```python
from build123d import *

# Parameters (mm, degrees)
SKETCH_4_OUTSIDE_W        = 310.112
SKETCH_4_OUTSIDE_H        = 310.112
CUT_EXTRUDE_1_DEPTH       = 28
HOLE_WIZARD_1_D           = 9
HOLE_WIZARD_1_CBORE_D     = 15
HOLE_WIZARD_1_CBORE_DEPTH = 9
HOLE_WIZARD_M30_2_D       = 26.5
CHAMFER_1_SIZE            = 1


with BuildPart() as part:
    # 草图3 → 旋转1 (revolve)
    with BuildSketch(Plane.XY, mode=Mode.PRIVATE) as revolve_1_sk:
        Polygon((0, 0), (-28, 0), (-28, -4), (-40, -4), (-80, -12), (-120, -12), (-120, -28), (-81, -28), (-45, -24), (0, -24), align=None)
    revolve(revolve_1_sk.sketch.rotate(Axis((0, 0, 0), (0, -1, 0)), 270), axis=Axis((0, 0, 0), (0, -1, 0)))

    # 草图4 outside → 切除-拉伸1 (cut)
    with BuildSketch(Plane(origin=(0, 0, 0), x_dir=(1, 0, 0), z_dir=(0, 1, 0))):
        Rectangle(SKETCH_4_OUTSIDE_W, SKETCH_4_OUTSIDE_H)
        with BuildLine():
            Line((-18.406763831, 31.296320472), (-9.905, 119.590513733))
            ThreePointArc((-9.905, 119.590513733), (0, 120), (9.905, 119.590513733))
            Line((9.905, 119.590513733), (18.406763831, 31.296320472))
            ThreePointArc((18.406763831, 31.296320472), (20.246227355, 22.568533354), (23.974016609, 14.465356118))
            ThreePointArc((23.974016609, 14.465356118), (24.248711306, 14), (24.514374178, 13.529429355))
            ThreePointArc((24.514374178, 13.529429355), (29.668036888, 6.249480544), (36.306790489, 0.292564843))
            Line((36.306790489, 0.292564843), (108.520922945, -51.217275242))
            ThreePointArc((108.520922945, -51.217275242), (103.923048454, -60), (98.615922945, -68.373238491))
            Line((98.615922945, -68.373238491), (17.900026658, -31.588885314))
            ThreePointArc((17.900026658, -31.588885314), (9.421809533, -28.818013897), (0.540357568, -27.994785473))
            ThreePointArc((0.540357568, -27.994785473), (0, -28), (-0.540357568, -27.994785473))
            ThreePointArc((-0.540357568, -27.994785473), (-9.421809533, -28.818013897), (-17.900026658, -31.588885314))
            Line((-17.900026658, -31.588885314), (-98.615922945, -68.373238491))
            ThreePointArc((-98.615922945, -68.373238491), (-103.923048454, -60), (-108.520922945, -51.217275242))
            Line((-108.520922945, -51.217275242), (-36.306790489, 0.292564843))
            ThreePointArc((-36.306790489, 0.292564843), (-29.668036888, 6.249480544), (-24.514374178, 13.529429355))
            ThreePointArc((-24.514374178, 13.529429355), (-24.248711306, 14), (-23.974016609, 14.465356118))
            ThreePointArc((-23.974016609, 14.465356118), (-20.246227355, 22.568533354), (-18.406763831, 31.296320472))
        make_face(mode=Mode.SUBTRACT)
    extrude(amount=-CUT_EXTRUDE_1_DEPTH, mode=Mode.SUBTRACT)

    # 打孔尺寸(%根据)内六角圆柱头螺钉的类型1 (through all)
    with Locations(Plane(origin=(0, -24, -34), x_dir=(0, 0, -1), z_dir=(0, -1, 0))):
        with Locations((0, 0), (-51, 29.444863729), (-51, -29.444863729)):
            CounterBoreHole(HOLE_WIZARD_1_D / 2, HOLE_WIZARD_1_CBORE_D / 2, HOLE_WIZARD_1_CBORE_DEPTH)

    # M30 螺纹孔2 (through all)
    with Locations(Plane.ZX):
        with Locations((0, 0)):
            Hole(HOLE_WIZARD_M30_2_D / 2)

    # 倒角1
    chamfer_1_edges = [part.edges().sort_by_distance(p)[0] for p in [
        (-0.270191364, 0, 27.998696338),
        (0, 0, 13.25),
        (0, -24, 13.25),
        (0, -28, -120),
        (-103.923048454, -28, 60),
        (0, -12, -120),
        (-103.923048454, -12, 60),
        (103.923048454, -28, 60),
        (103.923048454, -12, 60),
    ]]
    chamfer(chamfer_1_edges, length=CHAMFER_1_SIZE)


solid = part.part
```
For this review, take the finished solid that the model builds, in its own axes (mm). A direction names the side the tool comes from. Coordinates: 2 decimals unless noted, no trailing zeros. Order: outer loops, then holes, each group sorted by start corner. A loop starts at its lowest first (then second) coordinate and runs counter-clockwise, first axis right, second up. Notation, with made-up numbers: (43, 83.25) - (80, 83.25) arc R10 ccw to (80, 93.25) - close; hole circle Ø8 at (56, 88). An arc over 180 degrees is marked (long way). Answer as a JSON object with one key per item and string values. Group by question number.
1. For faces 4 (the flat face through (-85, -12, 48)), 5 (the cylindrical face through (-9.299, -13.86, 28.793)), 6 (the flat face through (0, -15, -39)), list the 3-axis set-ups (+Z, -Z, +X, -X, +Y, -Y) from which the entire face can be reached by the end or side of a thin tool; tool diameter is ignored.
2. We need section C-C on x = -83. State the section outline as (y, z) points.
3. For probe 1 along Z at (x, y) = (-6, -15.25); probe 2 along X at (y, z) = (-18.5, 17); probe 3 along X at (y, z) = (-20.5, 2), list the stretches that pass through material, from the lowest coordinate up.
4. Clearance check with flat-ended pins moving along their axes: P1, Ø10.5, axis at x = -29.44, z = 17, coming from the -Y side; P2, Ø16.5, axis at x = 2.5, z = -33, coming from the -Y side; P3, Ø10, axis at y = -15, z = 24, coming from the +X side. State where each tip first meets the part, or that it passes through.
5. The part is to be moulded in two halves that separate along X. For faces 1 (the cylindrical face through (-20.286, -13.86, -22.45)), 2 (the flat face through (24.5, -15, 17.1)), 3 (the flat face through (-26.2, -4, 13.5)), say which applies: pulls with the +X half, pulls with the -X half, needs draft (parallel to the pull), parting line crosses it, or undercut.
6. We need section B-B on z = 17. Give the number of separate pieces and of enclosed holes in the cut face, then the cut area to 3 significant figures.
7. We need section A-A on y = -7. State the section outline as (x, z) points.
Final values:
{
 "1": {"face 4": "+Z, -X, +Y", "face 5": "+Z, +Y, -Y", "face 6": "-Y"},
 "2": {"outline": "(-28, 33.01) - (-12, 33.01) - (-12, 61.26) - (-28, 61.26) - close"},
 "3": {"probe 1": "-119.85 to -38.5, -29.5 to -11.81, 11.81 to 28.26", "probe 2": "-60.55 to -36.94, -21.94 to 21.94, 36.94 to 60.55", "probe 3": "-39.52 to -13.1, 13.1 to 39.52"},
 "4": {"P1": "y = -15", "P2": "y = -24", "P3": "x = 77.37"},
 "5": {"face 1": "pulls with the -X half", "face 2": "undercut", "face 3": "needs draft"},
 "6": {"separate pieces": "3", "enclosed holes": "0", "area": "2,060 mm²"},
 "7": {"outline": "(-53.66, 12.08) - (-36.31, -0.29) arc R40 cw to (-24.51, -13.53) arc R28 ccw to (-23.97, -14.47) arc R40 cw to (-18.41, -31.3) - (-16.36, -52.51) arc R55 ccw to (16.36, -52.51) - (18.41, -31.3) arc R40 cw to (23.97, -14.47) arc R28 ccw to (24.51, -13.53) arc R40 cw to (36.31, -0.29) - (53.66, 12.08) arc R55 ccw to (37.29, 40.43) - (17.9, 31.59) arc R40 cw to (0.54, 27.99) arc R28 ccw to (-0.54, 27.99) arc R40 cw to (-17.9, 31.59) - (-37.29, 40.43) arc R55 ccw to start; hole circle Ø9 at (-29.44, 17); hole circle Ø26.5 at (0, 0); hole circle Ø9 at (0, -34); hole circle Ø9 at (29.44, 17)"}
}
